from build123d import *

# Parameters (mm, degrees)
ESQUISSE1_W        = 258
ESQUISSE1_H        = 148
ESQUISSE1_R        = 3
BOSS_EXTRU_2_DEPTH = 40


with BuildPart() as part:
    # Esquisse1 → Boss.-Extru.2 (new body)
    with BuildSketch(Plane.XY):
        Rectangle(ESQUISSE1_W, ESQUISSE1_H)
        with Locations((-121.832077187, -66.832077187)):
            Circle(ESQUISSE1_R, mode=Mode.SUBTRACT)
        with Locations((-121.832077187, 66.832077187)):
            Circle(ESQUISSE1_R, mode=Mode.SUBTRACT)
        with Locations((121.832077187, -66.832077187)):
            Circle(ESQUISSE1_R, mode=Mode.SUBTRACT)
        with Locations((121.832077187, 66.832077187)):
            Circle(ESQUISSE1_R, mode=Mode.SUBTRACT)
        Polygon((-111, -70), (111, -70), (125, -56), (125, 56), (111, 70), (-111, 70), (-125, 56), (-125, -56), align=None, mode=Mode.SUBTRACT)
    extrude(amount=BOSS_EXTRU_2_DEPTH)


solid = part.part
Read the model definition and answer for the solid it produces. Units are mm, in the model's axes. A direction names the side the tool comes from. Round coordinates to 2 decimals unless told otherwise and drop trailing zeros. Loops run counter-clockwise (first coordinate to the right, second up) from the corner with the lowest first, then second, coordinate; pieces in that order, holes last.
Q1. Section C-C on z = 37.5 is taken. Write down the section's boundary in (x, y).
Q2. Determine the mould class of faces 3 (the face through (-10, 72, 40)), 4 (the face through (-2, -70, 20)), 5 (the face through (-129, -1, 20)), 6 (the face through (119.62, 68.86, 19.72)) for opening direction X: released by +X, released by -X, zero draft, split by the parting line, or undercut.
Q3. Consider probe 1 along X at (y, z) = (-26, 21); probe 2 along Y at (x, z) = (7, 23); probe 3 along Y at (x, z) = (117.5, 6.5). Determine where each line is inside the solid, lowest interval first.
Q4. Section A-A on x = -24 is taken. Write down the section's boundary in (y, z), and give its area (3 significant figures).
Q5. This flat-tipped pin is pushed along its axis until it touches: pin 1 (3.5 mm diameter, centred on x = -121.83, y = -66.83, fed in from -Z). Where does it stop, or does it pass through?
Q6. Section B-B on y = -16 is taken. Write down the section's boundary in (x, z).
Q7. Which of the six approach directions +Z, -Z, +X, -X, +Y, -Y give full straight-line access (tool end or side, diameter ignored) to faces 1 (the face through (-2, -74, 20)), 2 (the face through (125, -1, 20))?
Output:
1. outline: (-129, -74) - (129, -74) - (129, 74) - (-129, 74) - close; hole (-125, -56) - (-111, -70) - (111, -70) - (125, -56) - (125, 56) - (111, 70) - (-111, 70) - (-125, 56) - close; hole circle Ø6 at (-121.83, -66.83); hole circle Ø6 at (-121.83, 66.83); hole circle Ø6 at (121.83, -66.83); hole circle Ø6 at (121.83, 66.83)
2. face 3: zero draft
2. face 4: undercut
2. face 5: released by -X
2. face 6: undercut
3. probe 1: x = -129 to -125, 125 to 129
3. probe 2: y = -74 to -70, 70 to 74
3. probe 3: y = -74 to -63.5, 63.5 to 74
4. outline: (-74, 0) - (-70, 0) - (-70, 40) - (-74, 40) - close; (70, 0) - (74, 0) - (74, 40) - (70, 40) - close
4. area: 320 mm2
5. pin 1: passes through
6. outline: (-129, 0) - (-125, 0) - (-125, 40) - (-129, 40) - close; (125, 0) - (129, 0) - (129, 40) - (125, 40) - close
7. face 1: +Z, -Z, +X, -X, -Y
7. face 2: +Z, -Z
